from build123d import *

# Parameters (mm, degrees)
SKETCH1_W                                           = 115
SKETCH1_H                                           = 45
BOSS_EXTRUDE1_DEPTH                                 = 5
CUT_EXTRUDE1_REACH                                  = 119.287
SKETCH2_R                                           = 9.8171
CSK_FOR_M2_COUNTERSUNK_FLAT_HEAD_SCREW1_D           = 2.4
CSK_FOR_M2_COUNTERSUNK_FLAT_HEAD_SCREW1_CSINK_D     = 5.4
CSK_FOR_M2_COUNTERSUNK_FLAT_HEAD_SCREW1_CSINK_ANGLE = 90
SKETCH13_W                                          = 52
SKETCH13_H                                          = 45
BOSS_EXTRUDE4_DEPTH                                 = 6
CHAMFER2_SIZE                                       = 6
M3_TAPPED_HOLE1_D                                   = 2.5
CHAMFER1_SIZE                                       = 3
SKETCH14_W                                          = 12.5
SKETCH14_H                                          = 30
BOSS_EXTRUDE5_DEPTH                                 = 5
BOSS_EXTRUDE6_DEPTH                                 = 5
FILLET1_R                                           = 2
CSK_FOR_M2_COUNTERSUNK_FLAT_HEAD_SCREW2_D           = 2.4
CSK_FOR_M2_COUNTERSUNK_FLAT_HEAD_SCREW2_DEPTH       = 5
CSK_FOR_M2_COUNTERSUNK_FLAT_HEAD_SCREW2_CSINK_D     = 5.4
CSK_FOR_M2_COUNTERSUNK_FLAT_HEAD_SCREW2_CSINK_ANGLE = 90
CSK_FOR_M2_COUNTERSUNK_FLAT_HEAD_SCREW2_TIP         = 0.721032743


with BuildPart() as part:
    # Sketch1 → Boss-Extrude1 (new body)
    with BuildSketch(Plane(origin=(0, 0, 0), x_dir=(1, 0, 0), z_dir=(0, 1, 0))):
        with Locations((57.5, 0)):
            Rectangle(SKETCH1_W, SKETCH1_H)
    extrude(amount=BOSS_EXTRUDE1_DEPTH)

    # Sketch2 → Cut-Extrude1 (cut, up to next)
    with BuildSketch(Plane(origin=(0, 5, 0), x_dir=(1, 0, 0), z_dir=(0, 1, 0)), mode=Mode.PRIVATE) as cut_extrude1_sk1:
        with Locations(Location((22.5, 0, 0), (0, 0, 270))):
            Circle(SKETCH2_R)
    cut_extrude1_tool1 = extrude(cut_extrude1_sk1.sketch, amount=-CUT_EXTRUDE1_REACH, mode=Mode.PRIVATE) & part.part
    add(cut_extrude1_tool1.solids().sort_by_distance((22.5, 5, 0))[0], mode=Mode.SUBTRACT)

    # CSK for M2 Countersunk Flat Head Screw1 (through all)
    with Locations(Plane(origin=(0, 5, 0), x_dir=(1, 0, 0), z_dir=(0, 1, 0))):
        with Locations((4, -18.5), (41, -18.5), (41, 5), (4, 5)):
            CounterSinkHole(CSK_FOR_M2_COUNTERSUNK_FLAT_HEAD_SCREW1_D / 2, CSK_FOR_M2_COUNTERSUNK_FLAT_HEAD_SCREW1_CSINK_D / 2, counter_sink_angle=CSK_FOR_M2_COUNTERSUNK_FLAT_HEAD_SCREW1_CSINK_ANGLE)

    # Sketch13 → Boss-Extrude4 (add)
    with BuildSketch(Plane(origin=(0, 5, 0), x_dir=(1, 0, 0), z_dir=(0, 1, 0))):
        with Locations((89, 0)):
            Rectangle(SKETCH13_W, SKETCH13_H)
    extrude(amount=BOSS_EXTRUDE4_DEPTH)

    # Chamfer2
    chamfer2_edges = [part.edges().sort_by_distance(p)[0] for p in [
        (63, 11, 0),
    ]]
    chamfer(chamfer2_edges, length=CHAMFER2_SIZE - 0.0001)  # a hair under: the kernel refuses the full size

    # M3 Tapped Hole1 (through all)
    with Locations(Plane(origin=(0, 11, 0), x_dir=(1, 0, 0), z_dir=(0, 1, 0))):
        with Locations((83, 16), (111, 16), (83, -16), (111, -16)):
            Hole(M3_TAPPED_HOLE1_D / 2)

    # Chamfer1
    chamfer1_edges = [part.edges().sort_by_distance(p)[0] for p in [
        (115, 5.5, -22.5),
        (115, 5.5, 22.5),
    ]]
    chamfer(chamfer1_edges, length=CHAMFER1_SIZE)

    # Sketch14 → Boss-Extrude5 (add)
    with BuildSketch(Plane(origin=(0, 0, 0), x_dir=(1, 0, 0), z_dir=(0, 1, 0))):
        with Locations((-6.25, 0)):
            Rectangle(SKETCH14_W, SKETCH14_H)
    extrude(amount=BOSS_EXTRUDE5_DEPTH)

    # Sketch17 → Boss-Extrude6 (add)
    with BuildSketch(Plane(origin=(0, 0, 0), x_dir=(1, 0, 0), z_dir=(0, 1, 0))):
        Polygon((-12.5, 15), (-12.5, 32.5), (55, 32.5), (55, 22.5), (0, 22.5), (0, 15), align=None)
        Polygon((-12.5, -15), (-12.5, -32.5), (55, -32.5), (55, -22.5), (0, -22.5), (0, -15), align=None)
    extrude(amount=BOSS_EXTRUDE6_DEPTH)

    # Fillet1
    fillet1_edges = [part.edges().sort_by_distance(p)[0] for p in [
        (55, 2.5, -22.5),
        (55, 2.5, -32.5),
        (-12.5, 2.5, -32.5),
        (-12.5, 2.5, 32.5),
        (55, 2.5, 32.5),
        (55, 2.5, 22.5),
    ]]
    fillet(fillet1_edges, radius=FILLET1_R)

    # CSK for M2 Countersunk Flat Head Screw2
    with Locations(Plane(origin=(0, 0, 0), x_dir=(-1, 0, 0), z_dir=(0, -1, 0))):
        with Locations((1.5, 0), (8.5, -10), (8.5, 10), (8.5, -28.5), (-4, -28.5), (-16.5, -28.5), (-41.5, -28.5), (-41.5, 28.5), (-29, 28.5), (-16.5, 28.5), (-4, 28.5), (8.5, 28.5), (-29, -28.5)):
            CounterSinkHole(CSK_FOR_M2_COUNTERSUNK_FLAT_HEAD_SCREW2_D / 2, CSK_FOR_M2_COUNTERSUNK_FLAT_HEAD_SCREW2_CSINK_D / 2, depth=CSK_FOR_M2_COUNTERSUNK_FLAT_HEAD_SCREW2_DEPTH, counter_sink_angle=CSK_FOR_M2_COUNTERSUNK_FLAT_HEAD_SCREW2_CSINK_ANGLE)
            with Locations((0, 0, -(CSK_FOR_M2_COUNTERSUNK_FLAT_HEAD_SCREW2_DEPTH + CSK_FOR_M2_COUNTERSUNK_FLAT_HEAD_SCREW2_TIP / 2))):  # 118° drill point
                Cone(0, CSK_FOR_M2_COUNTERSUNK_FLAT_HEAD_SCREW2_D / 2, CSK_FOR_M2_COUNTERSUNK_FLAT_HEAD_SCREW2_TIP, mode=Mode.SUBTRACT)


solid = part.part
Could you check a few things on this model? Use its own coordinates, in mm. A direction names the side the tool comes from. Give positions to 0.01 mm unless a question says otherwise; leave off trailing zeros. Order: outer loops, then holes, each group sorted by start corner. A loop starts at its lowest first (then second) coordinate and runs counter-clockwise, first axis right, second up. Notation, with made-up numbers: (-34, -9) - (-24, -9) arc R21 cw to (-24, 30) - close; hole circle Ø2 at (5.5, 63.5). An arc over 180 degrees is marked (long way). One line per item, written item: value. Start each with the question number.
1. Imagine slicing it at A-A on x = -1.5. List the corners of the cut face in (y, z) for me.
2. Imagine slicing it at D-D on x = 83. List the corners of the cut face in (y, z) for me.
3. Imagine slicing it at B-B on z = -16. Give the number of separate pieces and of enclosed holes in the cut face, plus the area to 4 significant figures.
4. Thinking about a two-plate mould opening in X: for faces 1 (the face through (81.81, 5.42, -16.38)), 2 (the face through (21, 2, 32.5)), 3 (the face through (-12.5, 2, 0)), 4 (the face through (30.11, 3.27, 28.96)), which applies, +X half, -X half, draft (parallel to the pull), parting line (faces both ways), or undercut?
5. If I drill on probe 1 along Z at (x, y) = (4, 2); probe 2 along X at (y, z) = (2.5, -16); probe 3 along Z at (x, y) = (111, 7.25), over which ranges is the centre line in solid material (lowest first)?
6. For faces 5 (the face through (84, 5, 22.5)), 6 (the face through (4.26, 1.73, 19.67)), 7 (the face through (84, 5, -22.5)), 8 (the face through (34, 5, 0)), which set-ups out of +Z, -Z, +X, -X, +Y, -Y let a thin tool reach every point of the face, with its end or its side?
7. For P1, Ø4, axis at x = -1.5, z = 0, coming from the -Y side; P2, Ø2, axis at x = 56.5, z = 2, coming from the +Y side; P3, Ø5.5, axis at x = 85, y = 7.5, coming from the -Z side, each with a flat end and sliding along its axis, tell me the tip position at first contact or that it passes through.
Values:
1. outline: (0, -32.5) - (5, -32.5) - (5, -1.2) - (1.5, -1.2) - (0, -2.7) - close; (0, 2.7) - (1.5, 1.2) - (5, 1.2) - (5, 32.5) - (0, 32.5) - close
2. outline: (0, -22.5) - (11, -22.5) - (11, -17.25) - (0, -17.25) - close; (0, -14.75) - (11, -14.75) - (11, 14.75) - (0, 14.75) - close; (0, 17.25) - (11, 17.25) - (11, 22.5) - (0, 22.5) - close
3. separate pieces: 3
3. enclosed holes: 0
3. area: 876.5 mm²
4. face 1: undercut
4. face 2: draft
4. face 3: -X half
4. face 4: undercut
5. probe 1: -32.5 to -29.7, -27.3 to -6.2, -3.8 to 17.3, 19.7 to 27.3, 29.7 to 32.5
5. probe 2: -12.5 to 81.75, 84.25 to 109.75, 112.25 to 115
5. probe 3: -22.5 to -17.25, -14.75 to 14.75, 17.25 to 22.5
6. face 5: +Z, +X, +Y, -Y
6. face 6: +Y, -Y
6. face 7: -Z, +X, +Y, -Y
6. face 8: +Z, -Z, -X, +Y
7. P1: y = 0.7
7. P2: y = 5
7. P3: z = -22.5
